Here's how the part is built. I have some questions about the finished solid (model axes, mm). A direction names the side the tool comes from. Round coordinates to 2 decimals unless told otherwise and drop trailing zeros. Order: outer loops, then holes, each group sorted by start corner. A loop starts at its lowest first (then second) coordinate and runs counter-clockwise, first axis right, second up.
```python
from build123d import *

# Parameters (mm, degrees)
Y_KSEKLIK_EKSTR_ZYON1_DEPTH      = 82
RADYUS1_R                        = 12
IZIM5_R                          = 6
KES_EKSTR_ZYON3_DEPTH            = 107
Y_KSEKLIK_EKSTR_ZYON2_DEPTH      = 6
Y_KSEKLIK_EKSTR_ZYON2_DEPTH_BACK = 6


with BuildPart() as part:
    # Çizim1 → Yükseklik-Ekstrüzyon1 (new body)
    with BuildSketch(Plane.XY):
        with BuildLine():
            Line((-78.213413995, -40.838458766), (-66.213413995, -40.838458766))
            Line((-66.213413995, -40.838458766), (-66.213413995, -16.838458766))
            Line((-66.213413995, -16.838458766), (15.786586005, -16.838458766))
            Line((15.786586005, -16.838458766), (15.786586005, -40.838458766))
            Line((15.786586005, -40.838458766), (27.804920328, -40.838458766))
            Line((27.804920328, -40.838458766), (27.804920328, -6.613491809))
            ThreePointArc((27.804920328, -6.613491809), (31.367545227, 2.717167386), (40.242234758, 7.299021041))
            ThreePointArc((40.242234758, 7.299021041), (54.188175449, 14.499076785), (59.786586005, 29.161541234))
            Line((59.786586005, 29.161541234), (47.768251683, 29.161541234))
            ThreePointArc((47.768251683, 29.161541234), (37.786586005, 19.179875557), (27.804920328, 29.161541234))
            Line((27.804920328, 29.161541234), (15.786586005, 29.161541234))
            Line((15.786586005, 29.161541234), (15.786586005, 7.161541234))
            ThreePointArc((15.786586005, 7.161541234), (12.271867379, -1.32374014), (3.786586005, -4.838458766))
            Line((3.786586005, -4.838458766), (-78.213413995, -4.838458766))
            Line((-78.213413995, -4.838458766), (-78.213413995, -40.838458766))
        make_face()
    extrude(amount=Y_KSEKLIK_EKSTR_ZYON1_DEPTH)

    # Radyus1
    radyus1_edges = [part.edges().sort_by_distance(p)[0] for p in [
        (21.795753166, -40.838458766, 0),
        (-72.213413995, -40.838458766, 0),
        (21.795753166, -40.838458766, 82),
        (-72.213413995, -40.838458766, 82),
    ]]
    fillet(radyus1_edges, radius=RADYUS1_R)

    # Çizim5 → Kes-Ekstrüzyon3 (cut)
    with BuildSketch(Plane.ZY.offset(78.213413995)):
        with Locations((12, -28.838458766)):
            Circle(IZIM5_R)
        with Locations((70, -28.838458766)):
            Circle(IZIM5_R)
    extrude(amount=-KES_EKSTR_ZYON3_DEPTH, mode=Mode.SUBTRACT)

    # Çizim8 → Yükseklik-Ekstrüzyon2 (add, two sides: drawn at the far end of the back side and taken through both)
    with BuildSketch(Plane.XY.offset(41).offset(-Y_KSEKLIK_EKSTR_ZYON2_DEPTH_BACK)):
        with BuildLine():
            Line((15.786586005, 29.161541234), (-78.213413995, -4.838458766))
            Line((-78.213413995, -4.838458766), (3.786586005, -4.838458766))
            ThreePointArc((3.786586005, -4.838458766), (12.271867379, -1.32374014), (15.786586005, 7.161541234))
            Line((15.786586005, 7.161541234), (15.786586005, 29.161541234))
        make_face()
    extrude(amount=Y_KSEKLIK_EKSTR_ZYON2_DEPTH + Y_KSEKLIK_EKSTR_ZYON2_DEPTH_BACK)


solid = part.part
```
1. If we section it at A-A, the plane z = 39: Write out the boundary of the cut face in (x, y), and give its area (3 significant figures).
Evaluation:
outline: (-78.21, -40.84) - (-66.21, -40.84) - (-66.21, -16.84) - (15.79, -16.84) - (15.79, -40.84) - (27.8, -40.84) - (27.8, -6.61) arc R14 cw to (40.24, 7.3) arc R22 ccw to (59.79, 29.16) - (47.77, 29.16) arc R9.98 cw to (27.8, 29.16) - (15.79, 29.16) - (-78.21, -4.84) - close
area: 4,340 mm2
2. If we section it at B-B, the plane y = -25: Write out the boundary of the cut face in (x, z).
Evaluation:
outline: (-78.21, 0) - (-66.21, 0) - (-66.21, 7.39) - (-78.21, 7.39) - close; (-78.21, 16.61) - (-66.21, 16.61) - (-66.21, 65.39) - (-78.21, 65.39) - close; (-78.21, 74.61) - (-66.21, 74.61) - (-66.21, 82) - (-78.21, 82) - close; (15.79, 0) - (27.8, 0) - (27.8, 7.39) - (15.79, 7.39) - close; (15.79, 16.61) - (27.8, 16.61) - (27.8, 65.39) - (15.79, 65.39) - close; (15.79, 74.61) - (27.8, 74.61) - (27.8, 82) - (15.79, 82) - close
3. I'm going to push flat-ended pins straight in: P1, Ø15.5, axis at y = -28.84, z = 12, coming from the +X side; P2, Ø17.5, axis at y = 21.5, z = 72.5, coming from the -X side; P3, Ø2, axis at x = -53.5, z = 71, coming from the +Y side. Where does each tip first touch, or does it pass through?
Evaluation:
P1: stops at x = 27.8
P2: stops at x = 15.79
P3: stops at y = -4.84
4. If we section it at D-D, the plane x = -63.5: Write out the boundary of the cut face in (y, z).
Evaluation:
outline: (-16.84, 0) - (-4.84, 0) - (-4.84, 35) - (0.48, 35) - (0.48, 47) - (-4.84, 47) - (-4.84, 82) - (-16.84, 82) - close
5. If we section it at C-C, the plane z = 66: Write out the boundary of the cut face in (x, y), and give its area (3 significant figures).
Evaluation:
outline: (-78.21, -40.84) - (-66.21, -40.84) - (-66.21, -33.31) - (-78.21, -33.31) - close; (-78.21, -24.37) - (-66.21, -24.37) - (-66.21, -16.84) - (15.79, -16.84) - (15.79, -24.37) - (27.8, -24.37) - (27.8, -6.61) arc R14 cw to (40.24, 7.3) arc R22 ccw to (59.79, 29.16) - (47.77, 29.16) arc R9.98 cw to (27.8, 29.16) - (15.79, 29.16) - (15.79, 7.16) arc R12 cw to (3.79, -4.84) - (-78.21, -4.84) - close; (15.79, -40.84) - (27.8, -40.84) - (27.8, -33.31) - (15.79, -33.31) - close
area: 2,560 mm2
6. If we mould it in two halves opening along Y, with no side actions, what happens to faces 1 (the flat face through (-11, 5, 47)), 2 (the cylindrical face through (21.88, -37.42, 3.61)), 3 (the cylindrical face through (-72.297, -34.696, 10.699))? For each: released by +Y, released by -Y, zero draft, split by the parting line, or undercut.
Evaluation:
face 1: zero draft
face 2: released by -Y
face 3: undercut
7. I need wall thicknesses on probe 1 along Y at (x, z) = (-70.25, 12); probe 2 along X at (y, z) = (-37, 5.5); probe 3 along Y at (x, z) = (-30, 13). Which ranges of each line are inside material? Lowest first, please.
Evaluation:
probe 1: y = -40.84 to -34.84, -22.84 to -4.84
probe 2: x = -78.21 to -66.21, 15.79 to 27.8
probe 3: y = -16.84 to -4.84
8. On a 3-axis mill with a long thin cutter (end or side, diameter ignored), from which of +Z, -Z, +X, -X, +Y, -Y can I reach the whole of each face in a straight line? I mean faces 4 (the cylindrical face through (12.365, -1.23, 64.255)), 5 (the flat face through (15.787, 18, 17)), 6 (the flat face through (27.805, -24, 40)). Say none if no direction works.
Evaluation:
face 4: +Z, -X, +Y
face 5: -Z, -X, +Y
face 6: +Z, -Z, +X, -Y
